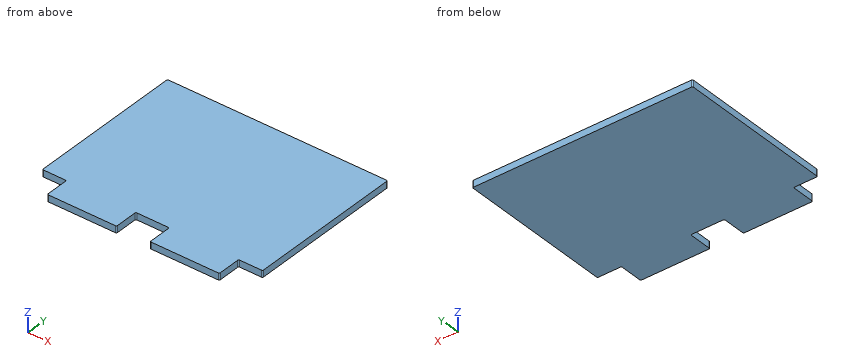
Autodesk Inventor part; units mm, degrees
sketch "Sketch1" plane through (0, 0, 0) normal (0, 0, 1) x (1, 0, 0)
  line L0 (-98.5, 80.75) -> (98.5, 80.75)
  line L1 (98.5, 80.75) -> (98.5, -80.75)
  line L2 (98.5, -80.75) -> (-98.5, -80.75)
  line L3 (-98.5, -80.75) -> (-98.5, 80.75)
  point P0 (0, 80.75)
  point P1 (0, 0)
  point P2 (-98.5, 0)
  dimension "d0" = 197
  dimension "d1" = 161.5
extrude "Extrusion1" add sketch "Sketch1" along normal blind 6
sketch "Sketch2" plane through (0, 0, 6) normal (0, 0, 1) x (1, 0, 0)
  line L0 (-98.5, 80.75) -> (-98.5, -80.75)
  line L1 (-98.5, -80.75) -> (-98.5, -59.25)
  line L2 (-98.5, -59.25) -> (-77, -59.25)
  line L3 (-98.5, -80.75) -> (98.5, -80.75)
  line L4 (-77, -59.25) -> (-77, -80.75)
  line L5 (-98.5, -80.75) -> (-77, -80.75)
  point P0 (0, 0)
  point P1 (40.5, -62.5)
  point P2 (-64.5, -80.75)
  dimension "d14" = 21.5
  dimension "d15" = 21.5
extrude "Extrusion2" cut sketch "Sketch2" against normal blind 15
mirror "Mirror1" about plane through (0, 0, 0) normal (1, 0, 0) of "Extrusion2"
sketch "Sketch4" plane through (0, 0, 6) normal (0, 0, 1) x (1, 0, 0)
  line L0 (-77, -80.75) -> (77, -80.75)
  line L1 (-15, -80.75) -> (15, -80.75)
  line L2 (15, -80.75) -> (15, -59.25)
  line L3 (15, -59.25) -> (-15, -59.25)
  line L4 (-15, -59.25) -> (-15, -80.75)
  point P0 (0, 0)
  point P1 (-64.5, -67.75)
  point P2 (64.5, -67.75)
  point P3 (0, -59.25)
  point P4 (0, -80.75)
  dimension "d18" = 30
  dimension "d19" = 21.5
extrude "Extrusion4" cut sketch "Sketch4" against normal blind 10
fillet "Fillet1" radius 1 12 edges at (-98.5, -59.25, 3) (-15, -80.75, 3) (15, -80.75, 3) (98.5, -59.25, 3) (-15, -59.25, 3) (15, -59.25, 3) (-98.5, 80.75, 3) (98.5, 80.75, 3) (-77, -59.25, 3) (-77, -80.75, 3) (77, -80.75, 3) (77, -59.25, 3)
equation "\"d7\" = d5"
properties part number "Side_Side_MDF" material "MDF Medium Density Fiberboard"
Part model, mm, in its own coordinate system. Round coordinates to 2 decimals unless told otherwise and drop trailing zeros. Order: outer loops, then holes, each group sorted by start corner. A loop starts at its lowest first (then second) coordinate and runs counter-clockwise, first axis right, second up. Notation, with made-up numbers: (58, -38) -> (97, -38) arc R16 cw to (97, -9) -> close; hole circle Ø3 at (-12, 33). An arc over 180 degrees is marked (long way). Put each result on its own line as item: value.
Q1. Band-saw the part on A-A (y = -64.5). Give the cut face in (x, z), and give its area (3 significant figures).
From the geometry:
outline: (-77, 0) -> (-15, 0) -> (-15, 6) -> (-77, 6) -> close; (15, 0) -> (77, 0) -> (77, 6) -> (15, 6) -> close
area: 744 mm2
Q2. Band-saw the part on B-B (z = 4). Give the cut face in (x, y), and give its area (3 significant figures).
From the geometry:
outline: (-98.5, -58.25) arc R1 ccw to (-97.5, -59.25) -> (-78, -59.25) arc R1 cw to (-77, -60.25) -> (-77, -79.75) arc R1 ccw to (-76, -80.75) -> (-16, -80.75) arc R1 ccw to (-15, -79.75) -> (-15, -60.25) arc R1 cw to (-14, -59.25) -> (14, -59.25) arc R1 cw to (15, -60.25) -> (15, -79.75) arc R1 ccw to (16, -80.75) -> (76, -80.75) arc R1 ccw to (77, -79.75) -> (77, -60.25) arc R1 cw to (78, -59.25) -> (97.5, -59.25) arc R1 ccw to (98.5, -58.25) -> (98.5, 79.75) arc R1 ccw to (97.5, 80.75) -> (-97.5, 80.75) arc R1 ccw to (-98.5, 79.75) -> close
area: 30,200 mm2
Q3. Wall check: line 1 (Y direction, x = -88.5, z = 5.1). Give the ranges that are in metal, low to high. Write a range as [from, to].
From the geometry:
line 1: y = [-59.25, 80.75]
Q4. Pin check, flat tips, straight feed: pin 1 Ø1.8 at (x, z) = (85, 2.5) entering from -Y; pin 2 Ø3 at (y, z) = (-68.5, 3.5) entering from +X; pin 3 Ø3 at (y, z) = (-65.5, 3) entering from -X. Stop position of each tip, or through.
From the geometry:
pin 1: stops at y = -59.25
pin 2: stops at x = 77
pin 3: stops at x = -77
Q5. Band-saw the part on C-C (x = 82.5). Give the cut face in (y, z), and give its area (3 significant figures).
From the geometry:
outline: (-59.25, 0) -> (80.75, 0) -> (80.75, 6) -> (-59.25, 6) -> close
area: 840 mm2
